```python
from build123d import *

# Parameters (mm, degrees)
BOSS_EXTRUDE1_DEPTH                             = 4
CUT_EXTRUDE4_DEPTH                              = 2.4
M3_CLEARANCE_HOLE1_D                            = 3.4
CSK_FOR_M3_FLAT_HEAD_MACHINE_SCREW1_D           = 3.4
CSK_FOR_M3_FLAT_HEAD_MACHINE_SCREW1_CSINK_D     = 6.3
CSK_FOR_M3_FLAT_HEAD_MACHINE_SCREW1_CSINK_ANGLE = 90
SKETCH11_W                                      = 17.5
SKETCH11_H                                      = 20
CUT_EXTRUDE3_DEPTH                              = 78.964735618
FILLET1_R                                       = 2
CSK_FOR_M3_FLAT_HEAD_MACHINE_SCREW2_D           = 3.4
CSK_FOR_M3_FLAT_HEAD_MACHINE_SCREW2_CSINK_D     = 6.3
CSK_FOR_M3_FLAT_HEAD_MACHINE_SCREW2_CSINK_ANGLE = 90
MOVE_FACE1_DEPTH                                = 4


# Read off the part's stored shape, not the designer's step: Move Face1
with BuildPart() as part:
    # Sketch2 → Boss-Extrude1 (new body)
    with BuildSketch(Plane.XY):
        Polygon((0, 57.5), (0, 0), (52.5, 0), (52.5, 51.5), (50.5, 51.5), (46.5, 55.5), (46.5, 57.5), align=None)
    extrude(amount=BOSS_EXTRUDE1_DEPTH)

    # Sketch12 → Cut-Extrude4 (cut)
    with BuildSketch(Plane.XY):
        Polygon((45, 41.766838493), (47.8, 43.383419246), (47.8, 46.616580754), (45, 48.233161507), (42.2, 46.616580754), (42.2, 43.383419246), align=None)
    extrude(amount=CUT_EXTRUDE4_DEPTH, mode=Mode.SUBTRACT)

    # M3 Clearance Hole1 (through all)
    with Locations(Plane.XY.offset(4)):
        with Locations((45, 45), (-45, 45), (-45, -45), (45, -45)):
            Hole(M3_CLEARANCE_HOLE1_D / 2)

    # CSK for M3 Flat Head Machine Screw1 (through all)
    with Locations(Plane.XY.offset(4)):
        with Locations((0, 40), (0, 0), (48, 0)):
            CounterSinkHole(CSK_FOR_M3_FLAT_HEAD_MACHINE_SCREW1_D / 2, CSK_FOR_M3_FLAT_HEAD_MACHINE_SCREW1_CSINK_D / 2, counter_sink_angle=CSK_FOR_M3_FLAT_HEAD_MACHINE_SCREW1_CSINK_ANGLE)

    # Sketch11 → Cut-Extrude3 (cut, through all)
    with BuildSketch(Plane.XY):
        with Locations((20.75, 28)):
            Rectangle(SKETCH11_W, SKETCH11_H)
    extrude(amount=CUT_EXTRUDE3_DEPTH, mode=Mode.SUBTRACT)

    # Fillet1
    fillet1_edges = [part.edges().sort_by_distance(p)[0] for p in [
        (29.5, 38, 2),
        (12, 38, 2),
        (12, 18, 2),
        (29.5, 18, 2),
    ]]
    fillet(fillet1_edges, radius=FILLET1_R)

    # CSK for M3 Flat Head Machine Screw2 (through all)
    with Locations(Plane(origin=(0, 0, 0), x_dir=(-1, 0, 0), z_dir=(0, 0, -1))):
        with Locations((-24, 54), (-40, 54)):
            CounterSinkHole(CSK_FOR_M3_FLAT_HEAD_MACHINE_SCREW2_D / 2, CSK_FOR_M3_FLAT_HEAD_MACHINE_SCREW2_CSINK_D / 2, counter_sink_angle=CSK_FOR_M3_FLAT_HEAD_MACHINE_SCREW2_CSINK_ANGLE)

    # Move Face1 outline → Move Face1 (cut)
    with BuildSketch(Plane.XY):
        Polygon((46.3, 55.417157288), (50.417157288, 51.3), (52.5, 51.3), (52.5, 51.5), (50.5, 51.5), (46.5, 55.5), (46.5, 57.5), (46.3, 57.5), align=None)
    extrude(amount=MOVE_FACE1_DEPTH, mode=Mode.SUBTRACT)

    # Mirror1: part across plane


with BuildPart() as part_1:
    add(part.part)
    add(part.part.mirror(Plane(origin=(0, 0, 0), x_dir=(0, 0, 1), z_dir=(0, -1, 0))))

    # Mirror2: part across plane


with BuildPart() as part_2:
    add(part_1.part)
    add(part_1.part.mirror(Plane(origin=(0, 0, 0), x_dir=(0, 0, 1), z_dir=(1, 0, 0))))


solid = part_2.part
```
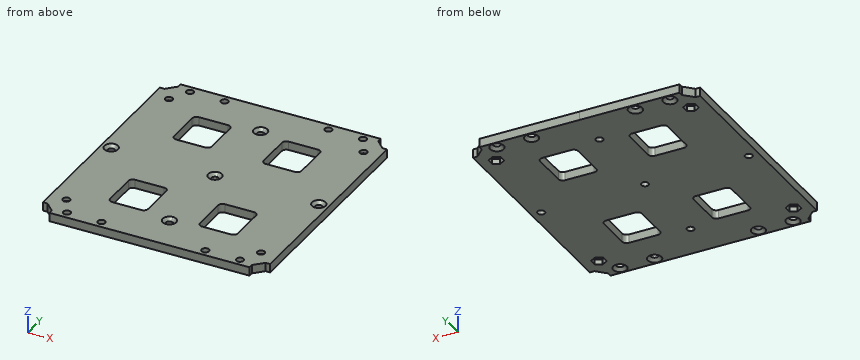
Check sheet for the modelled part. Datum: model origin and axes. Units: mm. Round coordinates to 2 decimals unless told otherwise and drop trailing zeros. Write each loop counter-clockwise with the first axis right and the second up, starting at its lowest first coordinate (ties: lowest second). Pieces come first, ordered by that corner, then holes. Notation, with made-up numbers: M 1,50.5 L 26,50.5 A22 cw 26,86.5 Z; hole C -23,-14.75 d11. An arc over 180 degrees is marked long. Write item = value, one per line. Start each with the question number.
1. Section check A-A, the plane y = -34.5. Record the cut outline in (x, z).
2. Section check D-D, the plane y = 54. Record the cut outline in (x, z).
3. Section check B-B, the plane x = -24. Record the cut outline in (y, z).
4. Section check C-C, the plane x = 40. Record the cut outline in (y, z).
5. Gauge pin test, flat ends, axial feed: pin 1 (4.5 mm diameter, centred on x = 24, y = -54, fed in from -Z); pin 2 (4 mm diameter, centred on x = -45, y = -45, fed in from -Z); pin 3 (1.7 mm diameter, centred on y = 56.5, z = 1, fed in from -X). Record the tip position at first contact, or that the pin passes through.
6. Scan lines: line 1 (X direction, y = -31.5, z = 3.7); line 2 (Y direction, x = 40, z = 2); line 3 (X direction, y = 0, z = 1). Record each from-to range of solid material in increasing order. Write a range as [from, to].
Results found:
q1.outline = M -52.5,0 L -29.5,0 L -29.5,4 L -52.5,4 Z; M -12,0 L 12,0 L 12,4 L -12,4 Z; M 29.5,0 L 52.5,0 L 52.5,4 L 29.5,4 Z
q2.outline = M -47.72,0 L -43.15,0 L -41.7,1.45 L -41.7,4 L -47.72,4 Z; M -38.3,1.45 L -36.85,0 L -27.15,0 L -25.7,1.45 L -25.7,4 L -38.3,4 Z; M -22.3,1.45 L -20.85,0 L 20.85,0 L 22.3,1.45 L 22.3,4 L -22.3,4 Z; M 25.7,1.45 L 27.15,0 L 36.85,0 L 38.3,1.45 L 38.3,4 L 25.7,4 Z; M 41.7,1.45 L 43.15,0 L 47.72,0 L 47.72,4 L 41.7,4 Z
q3.outline = M -57.5,0 L -57.15,0 L -55.7,1.45 L -55.7,4 L -57.5,4 Z; M -52.3,1.45 L -50.85,0 L -38,0 L -38,4 L -52.3,4 Z; M -18,0 L 18,0 L 18,4 L -18,4 Z; M 38,0 L 50.85,0 L 52.3,1.45 L 52.3,4 L 38,4 Z; M 55.7,1.45 L 57.15,0 L 57.5,0 L 57.5,4 L 55.7,4 Z
q4.outline = M -57.5,0 L -57.15,0 L -55.7,1.45 L -55.7,4 L -57.5,4 Z; M -52.3,1.45 L -50.85,0 L 50.85,0 L 52.3,1.45 L 52.3,4 L -52.3,4 Z; M 55.7,1.45 L 57.15,0 L 57.5,0 L 57.5,4 L 55.7,4 Z
q5.pin_1 = 0.9
q5.pin_2 = 2.4
q5.pin_3 = -46.3
q6.line_1 = [-52.5, -29.5], [-12, 12], [29.5, 52.5]
q6.line_2 = [-57.5, -55.7], [-52.3, 52.3], [55.7, 57.5]
q6.line_3 = [-52.5, -49.7], [-46.3, -1.7], [1.7, 46.3], [49.7, 52.5]
